For this review, use the dimensioned drawing (mm, ordinates from the lowest corner) and the shaded views. A direction names the side the tool comes from. Give positions to 0.01 mm unless a question says otherwise; leave off trailing zeros. Order: outer loops, then holes, each group sorted by start corner. A loop starts at its lowest first (then second) coordinate and runs counter-clockwise, first axis right, second up. Notation, with made-up numbers: M -27,64.5 L 15,64.5 A14 ccw 15,72.5 Z; hole C 47,47 d10. An arc over 180 degrees is marked long. One line per question, with ' | ' between items. Start each with the question number.
1. We need section D-D on x = 8. Write out the cut boundary in (y, z), then the cut area to 3 significant figures.
2. Insertion check: P1, Ø3, axis at x = 82.5, z = 15, coming from the -Y side; P2, Ø3, axis at y = 59.5, z = 13.5, coming from the +X side; P3, Ø2, axis at x = 22, z = 11, coming from the -Y side; P4, Ø3, axis at x = 90.5, z = 4, coming from the -Y side. Each pin has a flat end and moves straight along its axis. Give the tip position at first contact, or say it passes through.
3. Wall thickness on L1, parallel to Y at x = 57, z = 5.25; L2, parallel to X at y = 54, z = 16; L3, parallel to X at y = 33.5, z = 16: over which ranges is each line inside the solid? List them lowest first.
4. The part is to be moulded in two halves that separate along Y. For the marked faces 1, 2 and 3, say which applies: +Y half, -Y half, draft (parallel to the pull), parting line (faces both ways), or undercut.
5. For the marked faces 4, 5, 6, 7 and 8, list the 3-axis set-ups (+Z, -Z, +X, -X, +Y, -Y) from which the entire face can be reached by the end or side of a thin tool; tool diameter is ignored.
6. We need section A-A on y = 54. Write out the cut boundary in (x, z), then the cut area to 3 significant figures.
7. We need section C-C on x = 57. Write out the cut boundary in (y, z).
8. We need section B-B on z = 4. Write out the cut boundary in (x, y).
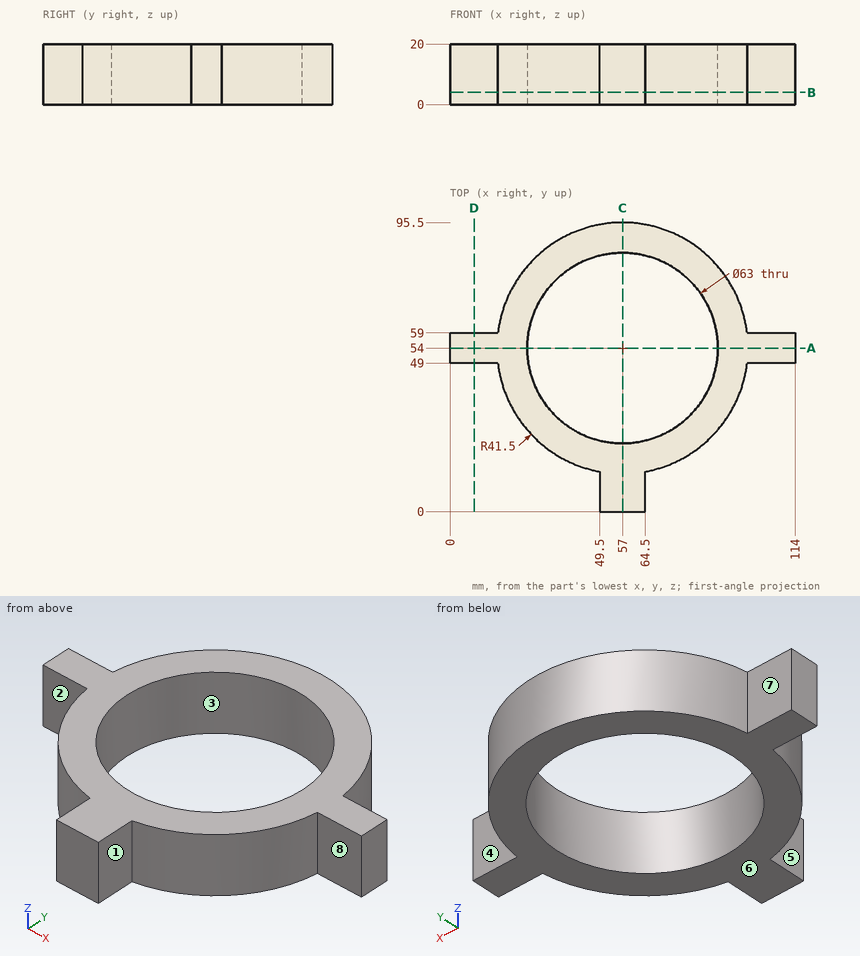
Entries:
1) outline: M 49,0 L 59,0 L 59,20 L 49,20 Z | area: 200 mm^2
2) P1: stops at y = 20.14 | P2: stops at x = 114 | P3: stops at y = 30.2 | P4: stops at y = 27.58
3) L1: y = 0 to 22.5, 85.5 to 95.5 | L2: x = 0 to 25.5, 88.5 to 114 | L3: x = 20.92 to 33.08, 80.92 to 93.08
4) face 1: draft | face 2: -Y half | face 3: undercut
5) face 4: +Z, -Z, +X, +Y | face 5: +Z, -Z, -X, -Y | face 6: -Z, +X, -X, +Y, -Y | face 7: +Z, -Z, -X, +Y | face 8: +Z, -Z, +X, -Y
6) outline: M 0,0 L 25.5,0 L 25.5,20 L 0,20 Z; M 88.5,0 L 114,0 L 114,20 L 88.5,20 Z | area: 1,020 mm^2
7) outline: M 0,0 L 22.5,0 L 22.5,20 L 0,20 Z; M 85.5,0 L 95.5,0 L 95.5,20 L 85.5,20 Z
8) outline: M 0,49 L 15.8,49 A41.5 ccw 49.5,13.18 L 49.5,0 L 64.5,0 L 64.5,13.18 A41.5 ccw 98.2,49 L 114,49 L 114,59 L 98.2,59 A41.5 ccw 15.8,59 L 0,59 Z; hole C 57,54 d63
